Can you work these out from the drawing? Everything is in mm from the part's minimum corner. A direction names the side the tool comes from. Coordinates: 2 decimals unless noted, no trailing zeros. Order: outer loops, then holes, each group sorted by start corner. A loop starts at its lowest first (then second) coordinate and runs counter-clockwise, first axis right, second up. Notation, with made-up numbers: (43.25, 61.25) - (69.25, 61.25) arc R25 ccw to (69.25, 76.25) - close; hole circle Ø4 at (47, 4). An arc over 180 degrees is marked (long way). One line per item, written item: value.
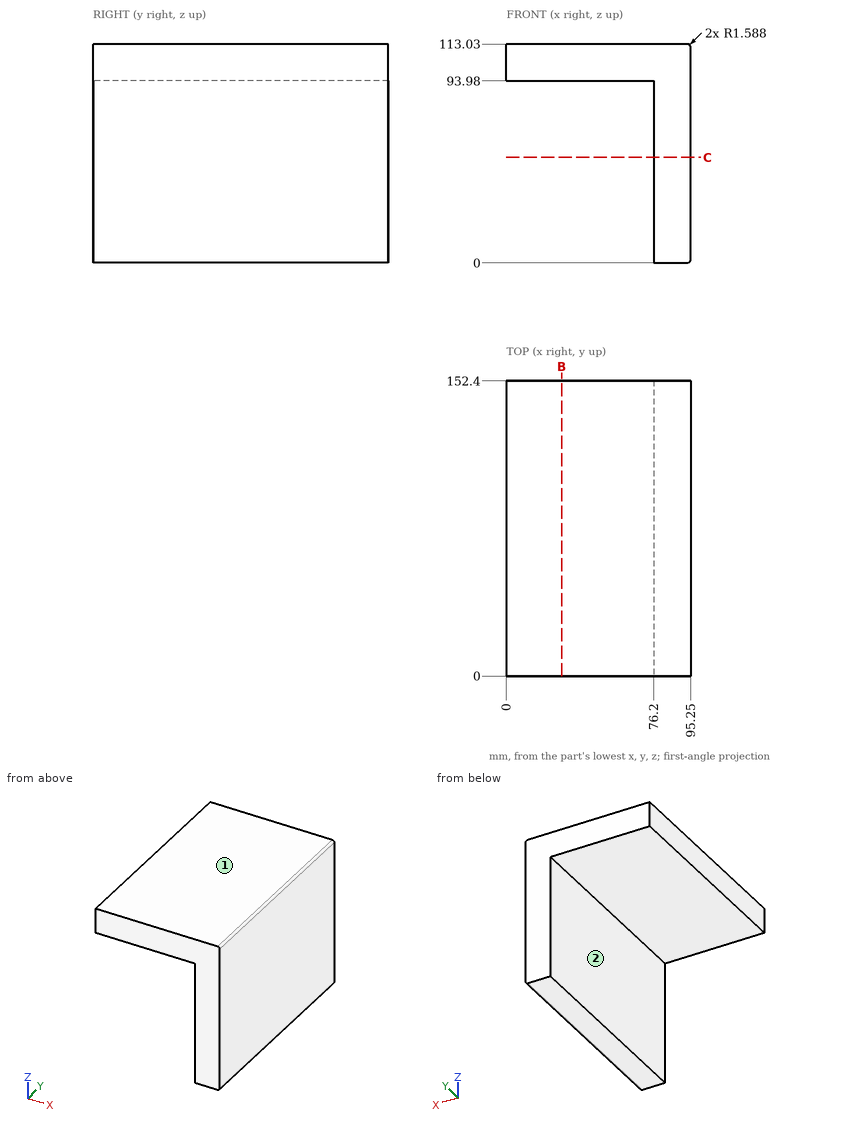
Item 1: I want a section at C-C on z = 54.5. Please give me the cut outline in (x, y), then the cut area to 3 significant figures.
Conclusion:
outline: (76.2, 0) - (95.25, 0) - (95.25, 152.4) - (76.2, 152.4) - close
area: 2,900 mm²
Item 2: For the marked faces 1 and 2, which set-ups out of +Z, -Z, +X, -X, +Y, -Y let a thin tool reach every point of the face, with its end or its side?
Conclusion:
face 1: +Z, +X, -X, +Y, -Y
face 2: -Z, -X, +Y, -Y
Item 3: I'm going to push a flat-ended pin straight in: pin 1 Ø6 at (y, z) = (50, 35) entering from -X. Where does the tip first touch, or does it pass through?
Conclusion:
pin 1: x = 76.2
Item 4: I want a section at B-B on x = 28.5. Please give me the cut outline in (y, z), then the cut area to 3 significant figures.
Conclusion:
outline: (0, 93.98) - (152.4, 93.98) - (152.4, 113.03) - (0, 113.03) - close
area: 2,900 mm²
Item 5: If I drill on probe 1 along X at (y, z) = (69, 20.5); probe 2 along Z at (x, y) = (14, 116.5), over which ranges is the centre line in solid material (lowest first)?
Conclusion:
probe 1: 76.2 to 95.25
probe 2: 93.98 to 113.03
